CAD build for the part. Positions are in the model's coordinates, mm. Face numbers are marked on the shaded views. A direction names the side the tool comes from. Give positions to 0.01 mm unless a question says otherwise; leave off trailing zeros. Write each loop counter-clockwise with the first axis right and the second up, starting at its lowest first coordinate (ties: lowest second). Pieces come first, ordered by that corner, then holes. Notation, with made-up numbers: (75.25, 51.5) - (91.25, 51.5) arc R16 cw to (91.25, 64.5) - close; hole circle Ø8 at (37.25, -8). An arc over 180 degrees is marked (long way). Answer as a JSON object with one key per item and string values.
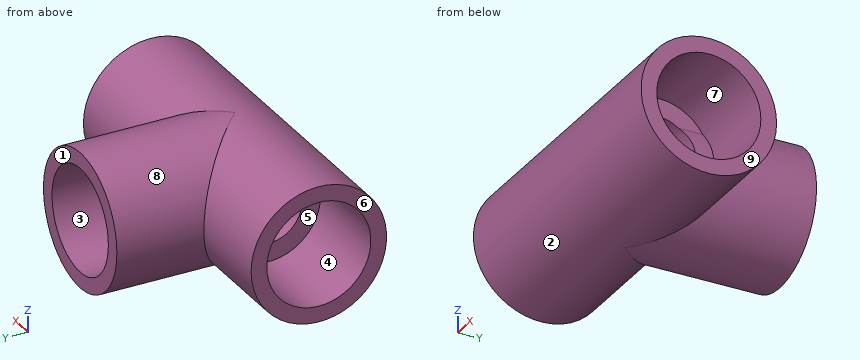
from build123d import *

# Parameters (mm, degrees)
SKETCH2_W               = 13.890625
SKETCH2_H               = 31.75
SKETCH4_R               = 6.9342
CUT_EXTRUDE1_DEPTH      = 32.7500001
CUT_EXTRUDE1_DEPTH_BACK = 32.7500001


with BuildPart() as part:
    # Sketch1 → Revolve1 (revolve)
    with BuildSketch(Plane.XY):
        Polygon((-31.75, 13.890625), (31.75, 13.890625), (31.75, 10.668), (12.7, 10.668), (12.7, 0), (-12.7, 0), (-12.7, 10.668), (-31.75, 10.668), align=None)
    revolve(axis=Axis((0, 0, 0), (1, 0, 0)))

    # Sketch2 → Revolve2 (revolve)
    with BuildSketch(Plane.XY):
        with Locations((-6.9453125, 15.875)):
            Rectangle(SKETCH2_W, SKETCH2_H)
    revolve(axis=Axis((0, 38.237555026, 0), (0, 1, 0)))

    # Sketch3 → Cut-Revolve1 (revolve, cut)
    with BuildSketch(Plane.XY):
        Polygon((0, 31.75), (-10.668, 31.75), (-10.668, 12.7), (-6.9342, 12.7), (-6.9342, 0), (0, 0), align=None)
    revolve(axis=Axis((0, 78.208657222, 0), (0, 1, 0)), mode=Mode.SUBTRACT)

    # Sketch4 → Cut-Extrude1 (cut, two sides)
    with BuildSketch(Plane(origin=(0, 0, 0), x_dir=(0, 0, -1), z_dir=(1, 0, 0))) as cut_extrude1_sk:
        Circle(SKETCH4_R)
    extrude(amount=CUT_EXTRUDE1_DEPTH, mode=Mode.SUBTRACT)
    extrude(cut_extrude1_sk.sketch, amount=-CUT_EXTRUDE1_DEPTH_BACK, mode=Mode.SUBTRACT)


solid = part.part
(1) Saw through at A-A, the plane z = 0. Give the cut face in (x, y), and give its area (3 significant figures).
Answer key:
{"outline": "(-31.75, -13.89) - (31.75, -13.89) - (31.75, -10.67) - (12.7, -10.67) - (12.7, -6.93) - (-12.7, -6.93) - (-12.7, -10.67) - (-31.75, -10.67) - close; (-31.75, 10.67) - (-13.89, 10.67) - (-13.89, 6.93) - (-6.93, 6.93) - (-6.93, 12.7) - (-10.67, 12.7) - (-10.67, 31.75) - (-13.89, 31.75) - (-13.89, 13.89) - (-31.75, 13.89) - close; (6.93, 6.93) - (13.89, 6.93) - (13.89, 10.67) - (31.75, 10.67) - (31.75, 13.89) - (13.89, 13.89) - (13.89, 31.75) - (10.67, 31.75) - (10.67, 12.7) - (6.93, 12.7) - close", "area": "618 mm²"}
(2) Saw through at B-B, the plane y = 5. Give the cut face in (x, z).
Answer key:
{"outline": "(-31.75, -12.96) - (-5, -12.96) arc R13.89 ccw to (5, -12.96) - (31.75, -12.96) - (31.75, -9.42) - (12.7, -9.42) - (12.7, -5.63) arc R13.89 ccw to (13.03, -4.8) - (5, -4.8) arc R6.93 cw to (-5, -4.8) - (-13.03, -4.8) arc R13.89 ccw to (-12.7, -5.63) - (-12.7, -9.42) - (-31.75, -9.42) - close; (-31.75, 9.42) - (-12.7, 9.42) - (-12.7, 5.63) arc R13.89 ccw to (-13.03, 4.8) - (-5, 4.8) arc R6.93 cw to (5, 4.8) - (13.03, 4.8) arc R13.89 ccw to (12.7, 5.63) - (12.7, 9.42) - (31.75, 9.42) - (31.75, 12.96) - (5, 12.96) arc R13.89 ccw to (-5, 12.96) - (-31.75, 12.96) - close"}
(3) Saw through at D-D, the plane x = -23.5. Give the cut face in (y, z), and give its area (3 significant figures).
Answer key:
{"outline": "circle Ø27.78 at (0, 0); hole circle Ø21.34 at (0, 0)", "area": "249 mm²"}
(4) Pull direction Y, two halves, no side cores. Call the marked faces 1, 2, 3 and 4: pulls with the +Y half, pulls with the -Y half, needs draft (parallel to the pull), parting line crosses it, or undercut.
Answer key:
{"face 1": "pulls with the +Y half", "face 2": "parting line crosses it", "face 3": "needs draft", "face 4": "undercut"}
(5) Saw through at C-C, the plane x = 0. Give the cut face in (y, z), and give its area (3 significant figures).
Answer key:
{"outline": "(0, -13.89) - (31.75, -13.89) - (31.75, -10.67) - (12.7, -10.67) - (12.7, -6.93) - (0, -6.93) arc R6.93 cw to (0, 6.93) - (12.7, 6.93) - (12.7, 10.67) - (31.75, 10.67) - (31.75, 13.89) - (0, 13.89) arc R13.89 ccw to start", "area": "527 mm²"}
(6) 3-axis set-ups, long thin cutter, end or side, ignore diameter. For the marked faces 5, 6, 7, 8 and 9: which of +Z, -Z, +X, -X, +Y, -Y reach the whole face in a straight line?
Answer key:
{"face 5": "-X", "face 6": "+Z, -Z, -X, +Y, -Y", "face 7": "+X", "face 8": "+Y", "face 9": "+Z, -Z, +X, +Y, -Y"}
(7) Flat gauge pins, fed straight in: P1, Ø5, axis at x = 9, y = -7, coming from the -Z side; P2, Ø1, axis at x = 8.5, y = 1, coming from the -Z side; P3, Ø3, axis at y = 15, z = 11, coming from the +X side. Where does each tip first touch, or does it go through?
Answer key:
{"P1": "stops at z = -13.14", "P2": "stops at z = -13.88", "P3": "stops at x = 10.13"}
(8) Probe L1, parallel to Z at x = 0, y = 5; L2, parallel to Y at x = 25.5, z = -0.5; L3, parallel to Z at x = 21.75, y = 0. List the from-to ranges inside material, lowest first. Write a range as [from, to].
Answer key:
{"L1": "z = [-13.89, -6.93], [6.93, 13.89]", "L2": "y = [-13.88, -10.66], [10.66, 13.88]", "L3": "z = [-13.89, -10.67], [10.67, 13.89]"}
